For this review, take the finished solid that the model builds, in its own axes (mm). Face numbers are marked on the shaded views. A direction names the side the tool comes from. Give positions to 0.01 mm unless a question says otherwise; leave off trailing zeros. Order: outer loops, then holes, each group sorted by start corner. A loop starts at its lowest first (then second) coordinate and runs counter-clockwise, first axis right, second up. Notation, with made-up numbers: (3.25, -30.5) -> (51.25, -30.5) arc R24 cw to (51.25, -15.5) -> close; hole circle Ø7 at (48.25, 19). An arc over 180 degrees is marked (long way). Return JSON: item names as keys, results as strings. Group by question number.
1) Add section A-A (y = 0). Give the boundary of the cut face in (x, z) (3 decimals), then the cut area to 3 significant figures.
2) The part is to be moulded in two halves that separate along Z. For the marked faces 1 and 2, say which applies: released by +Z, released by -Z, zero draft, split by the parting line, or undercut.
3) Add section D-D (y = -3.25). Give the boundary of the cut face in (x, z) (3 decimals), then the cut area to 3 significant figures.
4) Add section C-C (z = 13.5). Give the boundary of the cut face in (x, y).
5) For the marked faces 3 and 4, list the 3-axis set-ups (+Z, -Z, +X, -X, +Y, -Y) from which the entire face can be reached by the end or side of a thin tool; tool diameter is ignored.
6) Add section B-B (x = 15.25). Give the boundary of the cut face in (y, z) (3 decimals), then the cut area to 3 significant figures.
7) To check wall thickness, follow line 1 along Z through (x, y) = (13.5, -1.5) (3 decimals); line 2 along Z through (x, y) = (11.5, -4) (3 decimals); line 3 along Y through (x, z) = (18.75, 52). State the ranges of each line that lie inside material, in increasing order.
8) Insertion check: P1, Ø6, axis at y = 2.5, z = -9.5, coming from the +X side; P2, Ø6, axis at y = -3.5, z = 41.5, coming from the -X side; P3, Ø4, axis at y = -3, z = 31, coming from the -X side. Each pin has a flat end and moves straight along its axis. Give the tip position at first contact, or say it passes through.
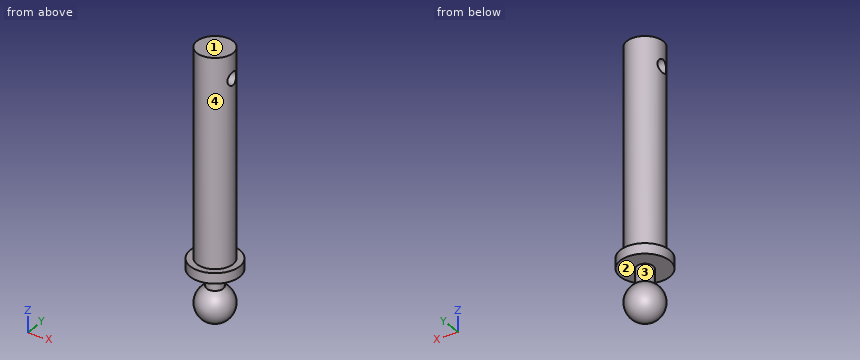
from build123d import *

# Parameters (mm, degrees)
RESSALTO_EXTRUS_O1_DEPTH      = 60
RESSALTO_EXTRUS_O1_DEPTH_BACK = 15
ESBO_O1_R                     = 5.497341607
CORTE_EXTRUS_O1_DEPTH         = 71
CORTE_EXTRUS_O1_DEPTH_BACK    = 71
ESBO_O2_R                     = 4
CORTE_EXTRUS_O3_DEPTH         = 64.97149057
CORTE_EXTRUS_O3_DEPTH_BACK    = 64.97149057
ESBO_O8_R                     = 2
RESSALTO_EXTRUS_O5_START      = -12
ESBO_O9_R                     = 7.5
RESSALTO_EXTRUS_O5_DEPTH      = 4
CORTE_EXTRUS_O5_DEPTH         = 65.872911801
ESBO_O12_R                    = 5.497341607
RESSALTO_EXTRUS_O6_DEPTH      = 3.5
ESBO_O14_R                    = 5.497341607
RESSALTO_EXTRUS_O7_DEPTH      = 6
CORTE_EXTRUS_O7_DEPTH         = 65.410749766
CORTE_EXTRUS_O7_DEPTH_BACK    = 65.410749766
ESBO_O16_R                    = 2
CORTE_EXTRUS_O8_DEPTH         = 65.410749766
CORTE_EXTRUS_O8_DEPTH_BACK    = 65.410749766
ESBO_O17_W                    = 10
ESBO_O17_H                    = 5.11854448
RESSALTO_EXTRUS_O8_START      = -14
RESSALTO_EXTRUS_O8_DEPTH      = 14
RESSALTO_EXTRUS_O9_START      = -1.79
RESSALTO_EXTRUS_O9_DEPTH      = 1.79
RESSALTO_EXTRUS_O10_DEPTH     = 2.21
ESBO_O21_R                    = 7.5
RESSALTO_EXTRUS_O11_DEPTH     = 3
CORTE_EXTRUS_O9_DEPTH         = 66.205232537
CORTE_EXTRUS_O9_DEPTH_BACK    = 66.205232537
ESBO_O22_W                    = 15
ESBO_O22_H                    = 25.435957471
ESBO_O23_R                    = 2.5
RESSALTO_EXTRUS_O12_DEPTH     = 10


with BuildPart() as part:
    # Esboço1 → Ressalto-extrusão1 (new, two sides: drawn at the far end of the back side and taken through both)
    with BuildSketch(Plane.XY.offset(-RESSALTO_EXTRUS_O1_DEPTH_BACK)):
        with Locations((15.99988667, 0)):
            Circle(ESBO_O1_R)
    extrude(amount=RESSALTO_EXTRUS_O1_DEPTH + RESSALTO_EXTRUS_O1_DEPTH_BACK)

    # Esboço2 → Corte-extrusão1 (cut, two sides: drawn at the far end of the back side and taken through both)
    with BuildSketch(Plane(origin=(0, 0, 0), x_dir=(0, 0, -1), z_dir=(1, 0, 0)).offset(-CORTE_EXTRUS_O1_DEPTH_BACK)):
        with Locations((-60, 0)):
            Circle(ESBO_O2_R)
    extrude(amount=CORTE_EXTRUS_O1_DEPTH + CORTE_EXTRUS_O1_DEPTH_BACK, mode=Mode.SUBTRACT)

    # Esboço8 → Corte-extrusão3 (cut, two sides: drawn at the far end of the back side and taken through both)
    with BuildSketch(Plane(origin=(0, 0, 0), x_dir=(0, 0, -1), z_dir=(1, 0, 0)).offset(-CORTE_EXTRUS_O3_DEPTH_BACK)):
        with Locations(Location((-52, 0, 0), (0, 0, 180))):
            Circle(ESBO_O8_R)
    extrude(amount=CORTE_EXTRUS_O3_DEPTH + CORTE_EXTRUS_O3_DEPTH_BACK, mode=Mode.SUBTRACT)

    # Esboço9 → Ressalto-extrusão5 (add)
    with BuildSketch(Plane(origin=(0, 0, -15), x_dir=(-1, 0, 0), z_dir=(0, 0, -1)).offset(RESSALTO_EXTRUS_O5_START)):
        with Locations((-15.99988667, 0)):
            Circle(ESBO_O9_R)
    extrude(amount=RESSALTO_EXTRUS_O5_DEPTH)

    # Esboço11 → Corte-extrusão5 (cut, through all)
    with BuildSketch(Plane(origin=(0, 0, 0), x_dir=(0, 0, -1), z_dir=(1, 0, 0))):
        Polygon((-56, -5.497341607), (-56, 0), (-56, 5.497341607), (-60, 5.497341607), (-60, 4), (-60, -5.497341607), align=None)
    extrude(amount=CORTE_EXTRUS_O5_DEPTH, mode=Mode.SUBTRACT)

    # Esboço12 → Ressalto-extrusão6 (add)
    with BuildSketch(Plane.XY.offset(56)):
        with Locations((15.99988667, 0)):
            Circle(ESBO_O12_R)
    extrude(amount=RESSALTO_EXTRUS_O6_DEPTH)

    # Esboço14 → Ressalto-extrusão7 (add)
    with BuildSketch(Plane(origin=(0, 0, -15), x_dir=(-1, 0, 0), z_dir=(0, 0, -1))):
        with Locations(Location((-15.99988667, 0, 0), (0, 0, 180))):
            Circle(ESBO_O14_R)
    extrude(amount=RESSALTO_EXTRUS_O7_DEPTH)

    # Esboço16 → Corte-extrusão7 (cut, two sides: drawn at the far end of the back side and taken through both)
    with BuildSketch(Plane(origin=(0, 0, 0), x_dir=(0, 0, -1), z_dir=(1, 0, 0)).offset(-CORTE_EXTRUS_O7_DEPTH_BACK)):
        with Locations((14.21, 0)):
            Circle(ESBO_O16_R)
    extrude(amount=CORTE_EXTRUS_O7_DEPTH + CORTE_EXTRUS_O7_DEPTH_BACK, mode=Mode.SUBTRACT)

    # Esboço17 → Corte-extrusão8 (cut, two sides: drawn at the far end of the back side and taken through both)
    with BuildSketch(Plane(origin=(0, 0, 0), x_dir=(0, 0, -1), z_dir=(1, 0, 0)).offset(-CORTE_EXTRUS_O8_DEPTH_BACK)):
        with Locations((14.21, -2.55927224)):
            Rectangle(ESBO_O17_W, ESBO_O17_H)
        with Locations((14.21, 2.55927224)):
            Rectangle(ESBO_O17_W, ESBO_O17_H)
    extrude(amount=CORTE_EXTRUS_O8_DEPTH + CORTE_EXTRUS_O8_DEPTH_BACK, mode=Mode.SUBTRACT)

    # Esboço18 → Ressalto-extrusão8 (add)
    with BuildSketch(Plane(origin=(0, 0, -21), x_dir=(-1, 0, 0), z_dir=(0, 0, -1)).offset(RESSALTO_EXTRUS_O8_START)):
        with BuildLine():
            Line((-21.481720524, 5.11854448), (-18.005196408, 5.11854448))
            ThreePointArc((-18.005196408, 5.11854448), (-15.99988667, 5.497341607), (-13.994576931, 5.11854448))
            Line((-13.994576931, 5.11854448), (-10.518052815, 5.11854448))
            ThreePointArc((-10.518052815, 5.11854448), (-15.99988667, 7.5), (-21.481720524, 5.11854448))
        make_face()
        with BuildLine():
            ThreePointArc((-13.994576931, -5.11854448), (-15.99988667, -5.497341607), (-18.005196408, -5.11854448))
            Line((-18.005196408, -5.11854448), (-21.481720524, -5.11854448))
            ThreePointArc((-21.481720524, -5.11854448), (-15.99988667, -7.5), (-10.518052815, -5.11854448))
            Line((-10.518052815, -5.11854448), (-13.994576931, -5.11854448))
        make_face()
    extrude(amount=RESSALTO_EXTRUS_O8_DEPTH)

    # Esboço19 → Ressalto-extrusão9 (add)
    with BuildSketch(Plane(origin=(0, 0, -21), x_dir=(-1, 0, 0), z_dir=(0, 0, -1)).offset(RESSALTO_EXTRUS_O9_START)):
        with BuildLine():
            ThreePointArc((-21.481720524, 5.11854448), (-23.49988667, 0), (-21.481720524, -5.11854448))
            Line((-21.481720524, -5.11854448), (-18.005196408, -5.11854448))
            ThreePointArc((-18.005196408, -5.11854448), (-21.497228276, 0), (-18.005196408, 5.11854448))
            Line((-18.005196408, 5.11854448), (-21.481720524, 5.11854448))
        make_face()
        with BuildLine():
            ThreePointArc((-10.518052815, -5.11854448), (-8.49988667, 0), (-10.518052815, 5.11854448))
            Line((-10.518052815, 5.11854448), (-13.994576931, 5.11854448))
            ThreePointArc((-13.994576931, 5.11854448), (-10.502545063, 0), (-13.994576931, -5.11854448))
            Line((-13.994576931, -5.11854448), (-10.518052815, -5.11854448))
        make_face()
    extrude(amount=RESSALTO_EXTRUS_O9_DEPTH)

    # Esboço20 → Ressalto-extrusão10 (add)
    with BuildSketch(Plane(origin=(0, 0, -7), x_dir=(-1, 0, 0), z_dir=(0, 0, -1))):
        with BuildLine():
            Line((-10.518052815, 5.11854448), (-13.994576931, 5.11854448))
            ThreePointArc((-13.994576931, 5.11854448), (-10.502545063, 0), (-13.994576931, -5.11854448))
            Line((-13.994576931, -5.11854448), (-10.518052815, -5.11854448))
            ThreePointArc((-10.518052815, -5.11854448), (-8.49988667, 0), (-10.518052815, 5.11854448))
        make_face()
        with BuildLine():
            Line((-18.005196408, 5.11854448), (-21.481720524, 5.11854448))
            ThreePointArc((-21.481720524, 5.11854448), (-23.49988667, 0), (-21.481720524, -5.11854448))
            Line((-21.481720524, -5.11854448), (-18.005196408, -5.11854448))
            ThreePointArc((-18.005196408, -5.11854448), (-21.497228276, 0), (-18.005196408, 5.11854448))
        make_face()
    extrude(amount=RESSALTO_EXTRUS_O10_DEPTH)

    # Esboço21 → Ressalto-extrusão11 (add)
    with BuildSketch(Plane(origin=(0, 0, -21), x_dir=(-1, 0, 0), z_dir=(0, 0, -1))):
        with Locations((-15.99988667, 0)):
            Circle(ESBO_O21_R)
    extrude(amount=RESSALTO_EXTRUS_O11_DEPTH)

    # Esboço22 → Corte-extrusão9 (cut, two sides: drawn at the far end of the back side and taken through both)
    with BuildSketch(Plane.XZ.offset(-5.11854448).offset(-CORTE_EXTRUS_O9_DEPTH_BACK)):
        with Locations((15.99988667, -18.822978736)):
            Rectangle(ESBO_O22_W, ESBO_O22_H)
    extrude(amount=CORTE_EXTRUS_O9_DEPTH + CORTE_EXTRUS_O9_DEPTH_BACK, mode=Mode.SUBTRACT)

    # Esboço23 → Ressalto-extrusão12 (add)
    with BuildSketch(Plane(origin=(0, 0, -6.105), x_dir=(-1, 0, 0), z_dir=(0, 0, -1))):
        with Locations(Location((-15.99988667, 0, 0), (0, 0, 90))):
            Circle(ESBO_O23_R)
    extrude(amount=RESSALTO_EXTRUS_O12_DEPTH)

    # Esboço24 → Revolução1 (revolve)
    with BuildSketch(Plane(origin=(0, 0, -16.105), x_dir=(-1, 0, 0), z_dir=(0, 0, -1))):
        with BuildLine():
            Line((-15.99988667, 5.497341607), (-15.99988667, -5.497341607))
            ThreePointArc((-15.99988667, -5.497341607), (-21.497228276, 0), (-15.99988667, 5.497341607))
        make_face()
    revolve(axis=Axis((15.99988667, 5.497341607, -16.105), (0, -1, 0)))


solid = part.part
Evaluation:
{
 "1": {"outline": "(8.5, -6.105) -> (13.5, -6.105) -> (13.5, -11.209) arc R5.497 ccw (long way) to (18.5, -11.209) -> (18.5, -6.105) -> (23.5, -6.105) -> (23.5, -3) -> (21.497, -3) -> (21.497, 50) -> (10.503, 50) -> (10.503, -3) -> (8.5, -3) -> close; (10.503, 54) -> (21.497, 54) -> (21.497, 59.5) -> (10.503, 59.5) -> close", "area": "808 mm^2"},
 "2": {"face 1": "released by +Z", "face 2": "undercut"},
 "3": {"outline": "(9.241, -6.105) -> (22.759, -6.105) -> (22.759, -3) -> (20.434, -3) -> (20.434, 59.5) -> (11.566, 59.5) -> (11.566, -3) -> (9.241, -3) -> close; circle Ø8.868 at (16, -16.105)", "area": "658 mm^2"},
 "4": {"outline": "circle Ø10.99 at (16, 0)"},
 "5": {"face 3": "none", "face 4": "+Z"},
 "6": {"outline": "(-7.462, -6.105) -> (-2.385, -6.105) -> (-2.385, -11.209) arc R5.446 ccw (long way) to (2.385, -11.209) -> (2.385, -6.105) -> (7.462, -6.105) -> (7.462, -3) -> (5.446, -3) -> (5.446, 59.5) -> (-5.446, 59.5) -> (-5.446, -3) -> (-7.462, -3) -> close; hole circle Ø4 at (0, 52)", "area": "830 mm^2"},
 "7": {"line 1": "-20.766 to -11.444, -6.105 to 50.677, 53.323 to 59.5", "line 2": "-6.105 to -3", "line 3": "-4.76 to -2, 2 to 4.76"},
 "8": {"P1": "x = 19.7", "P2": "x = 10.53", "P3": "x = 10.59"}
}
